Part model, mm, in its own coordinate system. A direction names the side the tool comes from. Give positions to 0.01 mm unless a question says otherwise; leave off trailing zeros. Loops run counter-clockwise (first coordinate to the right, second up) from the corner with the lowest first, then second, coordinate; pieces in that order, holes last. Notation, with made-up numbers: (-17, 50.5) -> (5, 50.5) arc R30 cw to (5, 80.5) -> close; hole circle Ø8 at (70.5, 76). An arc over 180 degrees is marked (long way). Write item = value, one per line.
from build123d import *

# Parameters (mm, degrees)
SKETCH1_R           = 22.5
BOSS_EXTRUDE1_DEPTH = 9
SKETCH2_R           = 2.25
CUT_EXTRUDE1_DEPTH  = 10
CIRPATTERN1_COUNT   = 4
SKETCH3_R           = 5
BOSS_EXTRUDE2_DEPTH = 18
CHAMFER1_SIZE       = 8
SKETCH6_R           = 10.75
CUT_EXTRUDE4_DEPTH  = 6


with BuildPart() as part:
    # Sketch1 → Boss-Extrude1 (new body)
    with BuildSketch(Plane(origin=(0, 0, 0), x_dir=(1, 0, 0), z_dir=(0, 1, 0))):
        Circle(SKETCH1_R)
    extrude(amount=BOSS_EXTRUDE1_DEPTH)

    # Sketch2 → Cut-Extrude1 (cut, through all)
    with BuildSketch(Plane(origin=(0, 9, 0), x_dir=(1, 0, 0), z_dir=(0, 1, 0))):
        with Locations((12.374368671, 12.374368671)):
            Circle(SKETCH2_R)
    cut_extrude1 = extrude(amount=-CUT_EXTRUDE1_DEPTH, mode=Mode.SUBTRACT)

    # CirPattern1: Cut-Extrude1 ×4 about axis
    cirpattern1_axis = Axis((0, 0, 0), (0, 1, 0))
    for i in range(1, CIRPATTERN1_COUNT):
        add(cut_extrude1.rotate(cirpattern1_axis, i * 360 / CIRPATTERN1_COUNT), mode=Mode.SUBTRACT)

    # Sketch3 → Boss-Extrude2 (add)
    with BuildSketch(Plane(origin=(0, 9, 0), x_dir=(1, 0, 0), z_dir=(0, 1, 0))):
        Circle(SKETCH3_R)
    extrude(amount=BOSS_EXTRUDE2_DEPTH)

    # Chamfer1
    chamfer1_edges = [part.edges().sort_by_distance(p)[0] for p in [
        (-5, 9, 0),
    ]]
    chamfer(chamfer1_edges, length=CHAMFER1_SIZE)

    # Sketch6 → Cut-Extrude4 (cut)
    with BuildSketch(Plane.XZ):
        Circle(SKETCH6_R)
    extrude(amount=-CUT_EXTRUDE4_DEPTH, mode=Mode.SUBTRACT)


solid = part.part
1) Which spindle directions (+Z, -Z, +X, -X, +Y, -Y) get a long thin tool onto all of the face, cutting with end or side? Do faces 1 (the face through (10.382, 4.437, 19.961)), 2 (the face through (10, 9, 10)), 3 (the face through (-1.4, 2.96, 10.66)). Say none if no direction does.
Resolved:
face_1 = +Y, -Y
face_2 = +Y
face_3 = -Y
2) Drill centre lines: line 1 along Y through (x, z) = (-13.5, -9.5); line 2 along Y through (x, z) = (-5, 2.5); line 3 along Z through (x, y) = (-1.5, 2). Where is each one in solid material? Low to high. Write a range as [from, to].
Resolved:
line_1 = [0, 9]
line_2 = [6, 16.41]
line_3 = [-22.45, -10.64], [10.64, 22.45]
3) Slice it at B-B, the plane z = 0. List the corners of the cut face in (x, y), and give its area (3 significant figures).
Resolved:
outline = (-22.5, 0) -> (-10.75, 0) -> (-10.75, 6) -> (10.75, 6) -> (10.75, 0) -> (22.5, 0) -> (22.5, 9) -> (13, 9) -> (5, 17) -> (5, 27) -> (-5, 27) -> (-5, 17) -> (-13, 9) -> (-22.5, 9) -> close
area = 520 mm²
4) Slice it at D-D, the plane y = 7.25. List the corners of the cut face in (x, z).
Resolved:
outline = circle Ø45 at (0, 0); hole circle Ø4.5 at (-12.37, -12.37); hole circle Ø4.5 at (-12.37, 12.37); hole circle Ø4.5 at (12.37, -12.37); hole circle Ø4.5 at (12.37, 12.37)
5) Slice it at C-C, the plane y = 16. List the corners of the cut face in (x, z).
Resolved:
outline = circle Ø12 at (0, 0)
6) Drop flat-ended pins along their axis: P1, Ø4, axis at x = -7, y = 14, coming from the -Z side; P2, Ø4, axis at x = 1, z = 6, coming from the -Y side; P3, Ø5, axis at y = 8, z = -2, coming from the +X side; P4, Ø1.5, axis at y = 6.5, z = 3, coming from the -X side. Give the stop position or say it passes through.
Resolved:
P1 = -7.66
P2 = 6
P3 = 22.5
P4 = -22.39
7) Slice it at A-A, the plane x = 0. List the corners of the cut face in (y, z), and give its area (3 significant figures).
Resolved:
outline = (0, -22.5) -> (9, -22.5) -> (9, -13) -> (17, -5) -> (27, -5) -> (27, 5) -> (17, 5) -> (9, 13) -> (9, 22.5) -> (0, 22.5) -> (0, 10.75) -> (6, 10.75) -> (6, -10.75) -> (0, -10.75) -> close
area = 520 mm²
8) Pull direction X, two halves, no side cores. Call faces 4 (the face through (-1.08, 21.93, 4.88)), 5 (the face through (0, 27, 0)), 6 (the face through (0, 6, 0)): pulls with the +X half, pulls with the -X half, needs draft (parallel to the pull), parting line crosses it, or undercut.
Resolved:
face_4 = parting line crosses it
face_5 = needs draft
face_6 = undercut
